```python
from build123d import *

# Parameters (mm, degrees)
SKETCH1_R           = 45
BOSS_EXTRUDE1_DEPTH = 9
SKETCH3_R           = 8.5
CUT_EXTRUDE2_DEPTH  = 10
SKETCH4_R           = 3
BOSS_EXTRUDE2_DEPTH = 6
SKETCH5_R           = 2.5
CUT_EXTRUDE3_DEPTH  = 5
CUT_EXTRUDE4_DEPTH  = 1


with BuildPart() as part:
    # Sketch1 → Boss-Extrude1 (new body)
    with BuildSketch(Plane(origin=(0, 0, 0), x_dir=(1, 0, 0), z_dir=(0, 1, 0))):
        with Locations(Location((0, 0, 0), (0, 0, 270))):
            Circle(SKETCH1_R)
    extrude(amount=BOSS_EXTRUDE1_DEPTH)

    # Sketch3 → Cut-Extrude2 (cut)
    with BuildSketch(Plane(origin=(0, 9, 0), x_dir=(1, 0, 0), z_dir=(0, 1, 0))):
        with Locations((0, 38.181883497)):
            Circle(SKETCH3_R)
    extrude(amount=-CUT_EXTRUDE2_DEPTH, mode=Mode.SUBTRACT)

    # Sketch4 → Boss-Extrude2 (add)
    with BuildSketch(Plane.XZ):
        with Locations(Location((0, 0, 0), (0, 0, 90))):
            Circle(SKETCH4_R)
    extrude(amount=BOSS_EXTRUDE2_DEPTH)

    # Sketch5 → Cut-Extrude3 (cut)
    with BuildSketch(Plane.XZ.offset(6)):
        with Locations(Location((0, 0, 0), (0, 0, 270))):
            Circle(SKETCH5_R)
    extrude(amount=-CUT_EXTRUDE3_DEPTH, mode=Mode.SUBTRACT)

    # Sketch6 → Cut-Extrude4 (cut)
    with BuildSketch(Plane(origin=(0, 9, 0), x_dir=(1, 0, 0), z_dir=(0, 1, 0))):
        with BuildLine():
            Line((-24.748737342, -24.748737342), (-28.284271247, -28.284271247))
            Line((-28.284271247, -28.284271247), (-30.405591591, -13.435028843))
            Line((-30.405591591, -13.435028843), (-15.556349186, -15.556349186))
            Line((-15.556349186, -15.556349186), (-19.091883092, -19.091883092))
            ThreePointArc((-19.091883092, -19.091883092), (-1.515e-06, -27), (19.09188095, -19.091885234))
            Line((19.09188095, -19.091885234), (15.556347044, -15.556351328))
            Line((15.556347044, -15.556351328), (30.405589449, -13.435030985))
            Line((30.405589449, -13.435030985), (28.284269105, -28.284273389))
            Line((28.284269105, -28.284273389), (24.7487352, -24.748739484))
            ThreePointArc((24.7487352, -24.748739484), (-1.515e-06, -35), (-24.748737342, -24.748737342))
        make_face()
    extrude(amount=-CUT_EXTRUDE4_DEPTH, mode=Mode.SUBTRACT)


solid = part.part
```
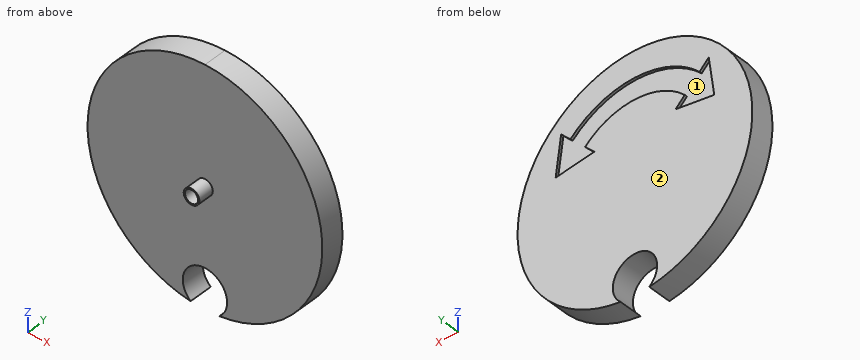
Check sheet for the modelled part. Datum: model origin and axes. Units: mm. Face numbers are marked on the shaded views. Coordinates: 2 decimals unless noted, no trailing zeros. Order: outer loops, then holes, each group sorted by start corner. A loop starts at its lowest first (then second) coordinate and runs counter-clockwise, first axis right, second up. Notation, with made-up numbers: M 3,-20.5 L 11,-20.5 A19 cw 11,5.5 Z; hole C 52.5,-4.75 d9. An arc over 180 degrees is marked long. Write each question's results on one line, items separated by ' | '. Start each with the question number.
1. Cross-section at A-A on z = 0. Record the cut outline in (x, y), and give its area (3 significant figures).
2. Mould release check, pull along Z, two halves, no side actions. Record for the marked faces 1 and 2: +Z half, -Z half, draft (parallel to the pull), parting line (faces both ways), or undercut.
3. Cross-section at D-D on x = -20.5. Record the cut outline in (y, z), and give its area (3 significant figures).
4. Cross-section at B-B on y = 5. Record the cut outline in (x, z), and give its area (3 significant figures).
5. Cross-section at C-C on x = 18. Record the cut outline in (y, z).
6. Go/stop test with flat-tipped pins: P1, Ø3, axis at x = 0, z = 0, coming from the -Y side; P2, Ø8, axis at x = -30.5, z = 34.5, coming from the -Y side; P3, Ø2, axis at y = 2.5, z = -16.5, coming from the +X side; P4, Ø4, axis at x = -1, z = -1, coming from the -Y side. Record where each tip stops, or that it passes through.
7. Material ranges on probe 1 along X at (y, z) = (-2.75, 0); probe 2 along Y at (x, z) = (-10.5, 20); probe 3 along Y at (x, z) = (-1.5, 28.5), recorded low to high.
Checks:
1) outline: M -45,0 L -3,0 L -3,-6 L -2.5,-6 L -2.5,-1 L 2.5,-1 L 2.5,-6 L 3,-6 L 3,0 L 45,0 L 45,9 L -45,9 Z | area: 821 mm²
2) face 1: undercut | face 2: draft
3) outline: M 0,-40.06 L 9,-40.06 L 9,14.85 L 8,14.85 L 8,28.37 L 9,28.37 L 9,40.06 L 0,40.06 Z | area: 708 mm²
4) outline: M -5.5,-44.66 A8.5 cw long 5.5,-44.66 A45 ccw long Z | area: 6,150 mm²
5) outline: M 0,-41.24 L 9,-41.24 L 9,15.21 L 8,15.21 L 8,18 L 9,18 L 9,20.12 L 8,20.12 L 8,30.02 L 9,30.02 L 9,41.24 L 0,41.24 Z
6) P1: stops at y = -1 | P2: stops at y = 0 | P3: stops at x = 42.25 | P4: stops at y = -6
7) probe 1: x = -3 to -2.5, 2.5 to 3 | probe 2: y = 0 to 9 | probe 3: y = 0 to 8
